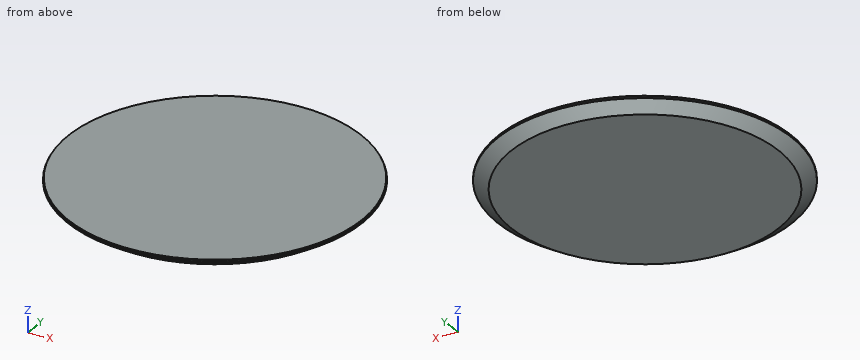
```python
from build123d import *

# Parameters (mm, degrees)
F0_R     = 22.05
F1_DEPTH = 1.5
F2_SIZE2 = 1.3
F2_SIZE  = 2
F3_R     = 21.95
F4_DEPTH = 0.2


with BuildPart() as f1:
    # F0 (on Top) → F1 (new body)
    with BuildSketch(Plane.XY):
        Circle(F0_R)
    extrude(amount=-F1_DEPTH)

    # F2
    f2_edges = [f1.edges().sort_by_distance(p)[0] for p in [
        (-22.05, 0, -1.5),
    ]]
    f2_side = f1.faces().sort_by_distance((0, 0, -1.5))[0]
    chamfer(f2_edges, length=F2_SIZE, length2=F2_SIZE2, reference=f2_side)

    # F3 (on face) → F4 (join)
    with BuildSketch(Plane.XY):
        Circle(F3_R)
    extrude(amount=F4_DEPTH)


solid = f1.part
```
For this review, take the finished solid that the model builds, in its own axes (mm). Round coordinates to 2 decimals unless told otherwise and drop trailing zeros. Order: outer loops, then holes, each group sorted by start corner. A loop starts at its lowest first (then second) coordinate and runs counter-clockwise, first axis right, second up.
Q1. Insertion check: P1, Ø1, axis at x = 11.5, z = -1.5, coming from the +Y side; P2, Ø1, axis at y = -5.5, z = 0, coming from the -X side. Each pin has a flat end and moves straight along its axis. Give the tip position at first contact, or say it passes through.
Findings below:
P1: stops at y = 17.41
P2: stops at x = -21.48
Q2. Wall thickness on line 1 (X direction, y = -9.5, z = -0.1); line 2 (Z direction, x = -18, y = -9); line 3 (X direction, y = -4, z = -0.8): over which ranges is each line inside the solid? List them lowest first.
Findings below:
line 1: x = -19.9 to 19.9
line 2: z = -1.45 to 0.2
line 3: x = -20.74 to 20.74
Q3. We need section A-A, the plane y = 0. Give the boundary of the cut face in (x, z), plus the area to 3 significant figures.
Findings below:
outline: (-22.05, -0.2) - (-20.05, -1.5) - (20.05, -1.5) - (22.05, -0.2) - (22.05, 0) - (21.95, 0) - (21.95, 0.2) - (-21.95, 0.2) - (-21.95, 0) - (-22.05, 0) - close
area: 72.3 mm2
Q4. We need section C-C, the plane z = -0.65. Give the boundary of the cut face in (x, y).
Findings below:
outline: circle Ø42.72 at (0, 0)
